Part model, mm, in its own coordinate system. Face numbers are marked on the shaded views. A direction names the side the tool comes from. Round coordinates to 2 decimals unless told otherwise and drop trailing zeros. Order: outer loops, then holes, each group sorted by start corner. A loop starts at its lowest first (then second) coordinate and runs counter-clockwise, first axis right, second up. Notation, with made-up numbers: M 26,-5 L 48,-5 A21 ccw 48,21 Z; hole C -1.5,-32 d3. An arc over 180 degrees is marked long. Write each question's results on one line, items separated by ' | '. Start each with the question number.
1. Band-saw the part on A-A, the plane z = 0. List the corners of the cut face in (x, y), then the cut area to 3 significant figures.
2. Band-saw the part on B-B, the plane y = 0. List the corners of the cut face in (x, z).
3. Drop flat-ended pins along their axis: pin 1 Ø6.5 at (x, y) = (-16.32, 0) entering from +Z; pin 2 Ø6 at (x, z) = (-24.5, 2) entering from +Y; pin 3 Ø8 at (y, z) = (2, -3.5) entering from -X; pin 4 Ø10 at (x, y) = (-16.5, 8.5) entering from -Z. Give the stop position or say it passes through.
4. Band-saw the part on D-D, the plane y = -4. List the corners of the cut face in (x, z).
5. Probe L1, parallel to X at y = 0, z = 7; L2, parallel to Y at x = -10, z = 0; L3, parallel to X at y = 2, z = 5.5. List the from-to ranges inside material, lowest first. Write a range as [from, to].
6. Two-plate mould, pull along X, no slides. Class the marked faces 1, 2 and 3: +X half, -X half, draft (parallel to the pull), parting line (faces both ways), or undercut.
7. Which spindle directions (+Z, -Z, +X, -X, +Y, -Y) get a long thin tool onto all of the face, cutting with end or side? Do the marked faces 4 and 5. Say none if no direction does.
8. Band-saw the part on C-C, the plane x = -17. List the corners of the cut face in (y, z), then the cut area to 3 significant figures.
```python
from build123d import *

# Parameters (mm, degrees)
CUT_EXTRUDE1_DEPTH      = 37.773634973
CUT_EXTRUDE1_DEPTH_BACK = 37.773634973
SKETCH2_R               = 2.5


with BuildPart() as part:
    # Sketch1 → Revolve1 (revolve)
    with BuildSketch(Plane.XY, mode=Mode.PRIVATE) as revolve1_sk:
        Polygon((-3.321167883, 11), (-6.321167883, 11), (-6.321167883, 10), (-33.321167883, 10), (-33.321167883, 5), (-3.321167883, 5), align=None)
    revolve(revolve1_sk.sketch.rotate(Axis((0, 0, 0), (-1, 0, 0)), 90), axis=Axis((0, 0, 0), (-1, 0, 0)))

    # Sketch2 → Cut-Extrude1 (cut, two sides: drawn at the far end of the back side and taken through both)
    with BuildSketch(Plane.XY.offset(-CUT_EXTRUDE1_DEPTH_BACK)):
        with Locations((-27.321167883, 0)):
            Circle(SKETCH2_R)
        with Locations((-16.321167883, 0)):
            Circle(SKETCH2_R)
    extrude(amount=CUT_EXTRUDE1_DEPTH + CUT_EXTRUDE1_DEPTH_BACK, mode=Mode.SUBTRACT)


solid = part.part
```
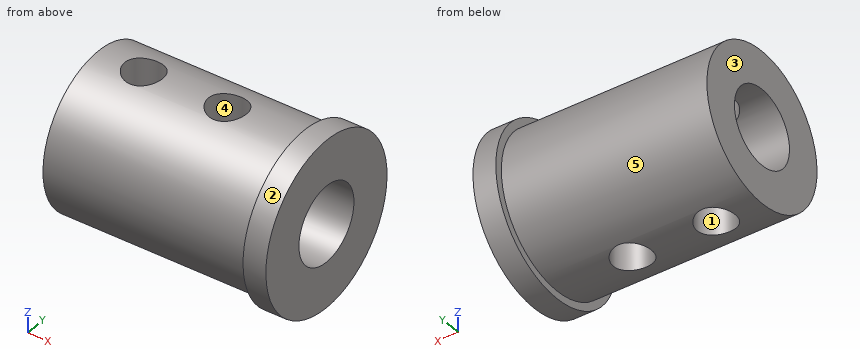
Solution:
1) outline: M -33.32,-10 L -6.32,-10 L -6.32,-11 L -3.32,-11 L -3.32,-5 L -33.32,-5 Z; M -33.32,5 L -3.32,5 L -3.32,11 L -6.32,11 L -6.32,10 L -33.32,10 Z | area: 306 mm^2
2) outline: M -33.32,-10 L -29.82,-10 L -29.82,-5 L -33.32,-5 Z; M -33.32,5 L -29.82,5 L -29.82,10 L -33.32,10 Z; M -24.82,-10 L -18.82,-10 L -18.82,-5 L -24.82,-5 Z; M -24.82,5 L -18.82,5 L -18.82,10 L -24.82,10 Z; M -13.82,-10 L -6.32,-10 L -6.32,-11 L -3.32,-11 L -3.32,-5 L -13.82,-5 Z; M -13.82,5 L -3.32,5 L -3.32,11 L -6.32,11 L -6.32,10 L -13.82,10 Z
3) pin 1: z = 10 | pin 2: y = 10 | pin 3: x = -33.32 | pin 4: z = -9.37
4) outline: M -33.32,-9.17 L -6.32,-9.17 L -6.32,-10.25 L -3.32,-10.25 L -3.32,-3 L -33.32,-3 Z; M -33.32,3 L -3.32,3 L -3.32,10.25 L -6.32,10.25 L -6.32,9.17 L -33.32,9.17 Z
5) L1: [-33.32, -29.82], [-24.82, -18.82], [-13.82, -3.32] | L2: [-10, -5], [5, 10] | L3: [-33.32, -28.82], [-25.82, -17.82], [-14.82, -3.32]
6) face 1: undercut | face 2: draft | face 3: -X half
7) face 4: +Z, -Z | face 5: -X
8) outline: M -2.41,-9.71 L -2.41,-4.38 A5 cw -2.41,4.38 L -2.41,9.71 A10 ccw Z; M 2.41,-9.71 A10 ccw 2.41,9.71 L 2.41,4.38 A5 cw 2.41,-4.38 Z | area: 187 mm^2
